Geometry: final body of the model. Coordinates: model frame, mm. Face numbers are marked on the shaded views. A direction names the side the tool comes from. Give positions to 0.01 mm unless a question says otherwise; leave off trailing zeros. Write each loop counter-clockwise with the first axis right and the second up, starting at its lowest first coordinate (ties: lowest second). Pieces come first, ordered by that corner, then holes. Notation, with made-up numbers: M -27.75,39.5 L -16.75,39.5 A21 cw -16.75,61.5 Z; hole C 1.25,25.25 d2. An arc over 180 degrees is marked long. One line per question, with ' | ' between items.
from build123d import *

# Parameters (mm, degrees)
SKETCH1_W           = 25
SKETCH1_H           = 25
SKETCH1_W_2         = 21
SKETCH1_H_2         = 21
BOSS_EXTRUDE1_DEPTH = 2
BOSS_EXTRUDE2_START = -2
SKETCH1_3_W         = 25
SKETCH1_3_H         = 25
SKETCH1_3_W_2       = 21
SKETCH1_3_H_2       = 21
BOSS_EXTRUDE2_DEPTH = 20
CUT_EXTRUDE1_REACH  = 37.57
SKETCH2_R           = 1.75
BOSS_EXTRUDE3_START = 12.5
BOSS_EXTRUDE3_DEPTH = 25
SKETCH4_R           = 3.3782
CUT_EXTRUDE2_DEPTH  = 44.259672441


with BuildPart() as part:
    # Sketch1 → Boss-Extrude1 (new body)
    # profile 1 of 2: a face of its own
    with BuildSketch(Plane(origin=(0, 0, 0), x_dir=(1, 0, 0), z_dir=(0, 1, 0))):
        Rectangle(SKETCH1_W, SKETCH1_H)
        Rectangle(SKETCH1_W_2, SKETCH1_H_2, mode=Mode.SUBTRACT)
    # profile 2 of 2: a face of its own
    with BuildSketch(Plane(origin=(0, 0, 0), x_dir=(1, 0, 0), z_dir=(0, 1, 0))):
        Rectangle(SKETCH1_W_2, SKETCH1_H_2)
    extrude(amount=-BOSS_EXTRUDE1_DEPTH)

    # Sketch1<3> → Boss-Extrude2 (add)
    with BuildSketch(Plane(origin=(0, 0, 0), x_dir=(1, 0, 0), z_dir=(0, 1, 0)).offset(BOSS_EXTRUDE2_START)):
        Rectangle(SKETCH1_3_W, SKETCH1_3_H)
        Rectangle(SKETCH1_3_W_2, SKETCH1_3_H_2, mode=Mode.SUBTRACT)
    extrude(amount=-BOSS_EXTRUDE2_DEPTH)

    # Sketch2 → Cut-Extrude1 (cut, up to next)
    with BuildSketch(Plane.XY.offset(-12.5), mode=Mode.PRIVATE) as cut_extrude1_sk1:
        with Locations(Location((0, -11, 0), (0, 0, 180))):
            Circle(SKETCH2_R)
    cut_extrude1_tool1 = extrude(cut_extrude1_sk1.sketch, amount=CUT_EXTRUDE1_REACH, mode=Mode.PRIVATE) & part.part
    add(cut_extrude1_tool1.solids().sort_by_distance((0, -11, -12.5))[0], mode=Mode.SUBTRACT)

    # Sketch3 → Boss-Extrude3 (add, through all)
    with BuildSketch(Plane(origin=(0, 0, 0), x_dir=(0, 0, -1), z_dir=(1, 0, 0)).offset(BOSS_EXTRUDE3_START)):
        Polygon((-12.5, 0), (-33.713203436, 21.213203436), (-30.17766953, 24.748737342), (-5.428932188, 0), align=None)
    extrude(amount=-BOSS_EXTRUDE3_DEPTH)

    # Sketch4 → Cut-Extrude2 (cut, through all)
    with BuildSketch(Plane(origin=(0, -6.25, 6.25), x_dir=(1, 0, 0), z_dir=(0, -0.7071067811865467, 0.7071067811865485))):
        with Locations(Location((0, 23.838834765, 0), (0, 0, 270))):
            Circle(SKETCH4_R)
    extrude(amount=-CUT_EXTRUDE2_DEPTH, mode=Mode.SUBTRACT)


solid = part.part
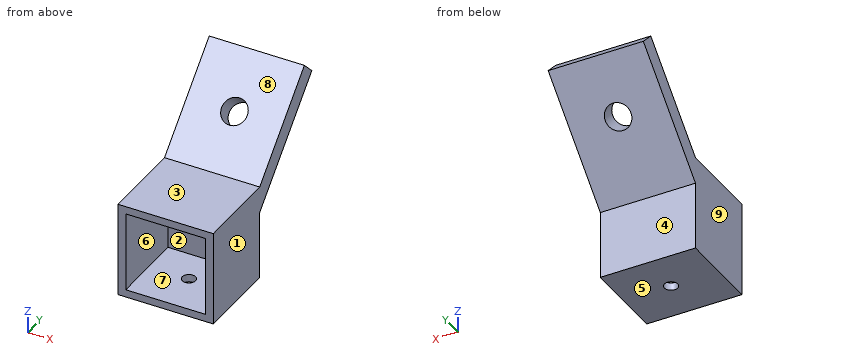
(1) Draft query along X for the marked faces 6, 7, 8 and 9. Return one class per face: released by +X, released by -X, zero draft, split by the parting line, or undercut.
Working result:
face 6: undercut | face 7: undercut | face 8: zero draft | face 9: released by -X
(2) First-contact query: P1, Ø10, axis at x = -7, y = 4, coming from the +Z side; P2, Ø2, axis at x = -2, z = 17, coming from the +Y side; P3, Ø1.5, axis at y = 17.5, z = 21.5, coming from the -X side; P4, Ø3, axis at x = 5, z = 17, coming from the +Y side. Flat tips, straight axial feed; report the tip coordinate or a pass-through.
Working result:
P1: stops at z = 21.5 | P2: stops at y = 12.48 | P3: passes through | P4: stops at y = 13.07
(3) Cut plane B-B, the plane y = -11. Return loops of the section in (x, z).
Working result:
outline: M -12.5,-12.5 L -1.75,-12.5 L -1.75,-10.5 L -10.5,-10.5 L -10.5,10.5 L 10.5,10.5 L 10.5,-10.5 L 1.75,-10.5 L 1.75,-12.5 L 12.5,-12.5 L 12.5,12.5 L -12.5,12.5 Z
(4) Cut plane D-D, the plane z = 14. Return loops of the section in (x, y).
Working result:
outline: M -12.5,1.5 L 12.5,1.5 L 12.5,8.57 L -12.5,8.57 Z
(5) Cut plane C-C, the plane x = 5. Return loops of the section in (y, z), then the cut area to 4 significant figures.
Working result:
outline: M -22,-12.5 L 0,-12.5 L 0,5.43 L 24.75,30.18 L 21.21,33.71 L 0,12.5 L -22,12.5 L -22,10.5 L -2,10.5 L -2,-10.5 L -22,-10.5 Z | area: 292.5 mm^2
(6) Cut plane A-A, the plane x = -1. Return loops of the section in (y, z).
Working result:
outline: M -22,-12.5 L -12.44,-12.5 L -12.44,-10.5 L -22,-10.5 Z; M -22,10.5 L -2,10.5 L -2,-10.5 L -9.56,-10.5 L -9.56,-12.5 L 0,-12.5 L 0,5.43 L 11.86,17.29 L 8.32,20.82 L 0,12.5 L -22,12.5 Z; M 12.89,25.39 L 16.42,21.85 L 24.75,30.18 L 21.21,33.71 Z
(7) Set-up query: the marked faces 1, 2, 3, 4 and 5. Return all of +Z, -Z, +X, -X, +Y, -Y with unobstructed straight access to the full face (end or side cutting, diameter ignored); none if empty.
Working result:
face 1: +Z, -Z, +X, +Y, -Y | face 2: -Y | face 3: +Z, +X, -X, -Y | face 4: -Z, +X, -X, +Y | face 5: -Z, +X, -X, +Y, -Y
(8) Material intervals for L1, parallel to X at y = -11, z = -11.65; L2, parallel to Z at x = -4, y = -9.5; L3, parallel to Y at x = 0, z = -11.15, sorted ascending. Write a range as [from, to].
Working result:
L1: x = [-12.5, -1.75], [1.75, 12.5] | L2: z = [-12.5, -10.5], [10.5, 12.5] | L3: y = [-22, -12.75], [-9.25, 0]
